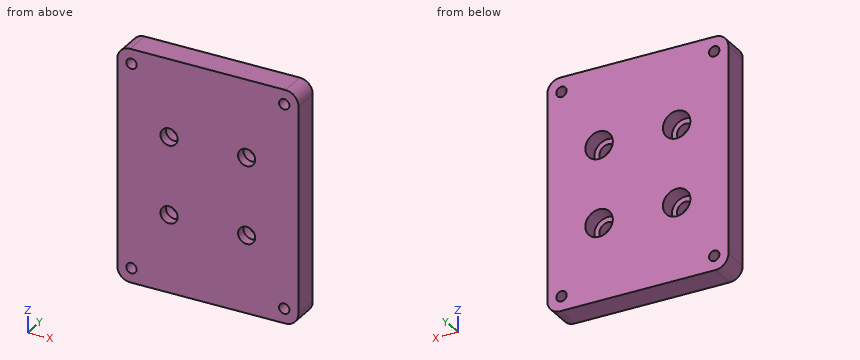
from build123d import *

# Parameters (mm, degrees)
SKETCH1_W                                         = 88.9
SKETCH1_H                                         = 114.3
BOSS_EXTRUDE1_DEPTH                               = 12.7
FILLET1_R                                         = 6.35
CBORE_FOR_5_16_SOCKET_HEAD_CAP_SCREW1_D           = 8.4328
CBORE_FOR_5_16_SOCKET_HEAD_CAP_SCREW1_CBORE_D     = 13.49502
CBORE_FOR_5_16_SOCKET_HEAD_CAP_SCREW1_CBORE_DEPTH = 7.9375
F_1_4_20_TAPPED_HOLE1_D                           = 5.1054


with BuildPart() as part:
    # Sketch1 → Boss-Extrude1 (new body)
    with BuildSketch(Plane(origin=(0, 0, 0), x_dir=(1, 0, 0), z_dir=(0, 1, 0))):
        Rectangle(SKETCH1_W, SKETCH1_H)
    extrude(amount=BOSS_EXTRUDE1_DEPTH)

    # Fillet1
    fillet1_edges = [part.edges().sort_by_distance(p)[0] for p in [
        (-44.45, 6.35, -57.15),
        (44.45, 6.35, -57.15),
        (44.45, 6.35, 57.15),
        (-44.45, 6.35, 57.15),
    ]]
    fillet(fillet1_edges, radius=FILLET1_R)

    # CBORE for 5/16 Socket Head Cap Screw1 (through all)
    with Locations(Plane(origin=(0, 12.7, 0), x_dir=(1, 0, 0), z_dir=(0, 1, 0))):
        with Locations((-19.05, 19.05), (-19.05, -19.05), (19.05, -19.05), (19.05, 19.05)):
            CounterBoreHole(CBORE_FOR_5_16_SOCKET_HEAD_CAP_SCREW1_D / 2, CBORE_FOR_5_16_SOCKET_HEAD_CAP_SCREW1_CBORE_D / 2, CBORE_FOR_5_16_SOCKET_HEAD_CAP_SCREW1_CBORE_DEPTH)

    # 1/4-20 Tapped Hole1 (through all)
    with Locations(Plane(origin=(0, 12.7, 0), x_dir=(1, 0, 0), z_dir=(0, 1, 0))):
        with Locations((-37.5, 50), (37.5, 50), (37.5, -50), (-37.5, -50)):
            Hole(F_1_4_20_TAPPED_HOLE1_D / 2)


solid = part.part
The listing builds one solid part. Answer for the finished solid, in the listing's coordinates (mm). Round coordinates to 2 decimals unless told otherwise and drop trailing zeros. Order: outer loops, then holes, each group sorted by start corner. A loop starts at its lowest first (then second) coordinate and runs counter-clockwise, first axis right, second up. Notation, with made-up numbers: (55, -7.5) -> (99, -7.5) arc R9 ccw to (99, 5.5) -> close; hole circle Ø6 at (-34.75, 53). An arc over 180 degrees is marked (long way). One line per item, written item: value.
Item 1: Straight lines are drawn through the part: L1, parallel to Z at x = 18.5, y = 6.25; L2, parallel to X at y = 10.5, z = -19.05; L3, parallel to X at y = 1.95, z = 19.05. For each, find the intervals that lie inside material, in ascending order.
Taken from the geometry:
L1: z = -57.15 to -25.78, -12.32 to 12.32, 25.78 to 57.15
L2: x = -44.45 to -25.8, -12.3 to 12.3, 25.8 to 44.45
L3: x = -44.45 to -23.27, -14.83 to 14.83, 23.27 to 44.45
Item 2: Find section A-A, the plane y = 3.5. State how many separate pieces and enclosed holes the cut face has, then the cut area to 3 significant figures.
Taken from the geometry:
separate pieces: 1
enclosed holes: 8
area: 9,820 mm2
Item 3: Find section C-C, the plane x = -19.05. Give the vertices of the cut face in (y, z), then the cut area to 3 significant figures.
Taken from the geometry:
outline: (0, -57.15) -> (12.7, -57.15) -> (12.7, -25.8) -> (4.76, -25.8) -> (4.76, -23.27) -> (0, -23.27) -> close; (0, -14.83) -> (4.76, -14.83) -> (4.76, -12.3) -> (12.7, -12.3) -> (12.7, 12.3) -> (4.76, 12.3) -> (4.76, 14.83) -> (0, 14.83) -> close; (0, 23.27) -> (4.76, 23.27) -> (4.76, 25.8) -> (12.7, 25.8) -> (12.7, 57.15) -> (0, 57.15) -> close
area: 1,160 mm2
Item 4: Find section B-B, the plane z = -19.05. Give the vertices of the cut face in (x, y).
Taken from the geometry:
outline: (-44.45, 0) -> (-23.27, 0) -> (-23.27, 4.76) -> (-25.8, 4.76) -> (-25.8, 12.7) -> (-44.45, 12.7) -> close; (-14.83, 0) -> (14.83, 0) -> (14.83, 4.76) -> (12.3, 4.76) -> (12.3, 12.7) -> (-12.3, 12.7) -> (-12.3, 4.76) -> (-14.83, 4.76) -> close; (23.27, 0) -> (44.45, 0) -> (44.45, 12.7) -> (25.8, 12.7) -> (25.8, 4.76) -> (23.27, 4.76) -> close
Item 5: Given P1, Ø6.5, axis at x = 19.05, z = -19.05, coming from the +Y side; P2, Ø4, axis at x = 19, z = 22, coming from the +Y side, each flat-ended and moving along its own axis, determine where each tip first touches the part or whether it passes through.
Taken from the geometry:
P1: passes through
P2: stops at y = 4.76
